Check sheet for the modelled part. Datum: model origin and axes. Units: mm. Face numbers are marked on the shaded views. A direction names the side the tool comes from. Give positions to 0.01 mm unless a question says otherwise; leave off trailing zeros. Order: outer loops, then holes, each group sorted by start corner. A loop starts at its lowest first (then second) coordinate and runs counter-clockwise, first axis right, second up. Notation, with made-up numbers: M 15,29 L 30,29 A27 ccw 30,62 Z; hole C 7,14 d2. An arc over 180 degrees is marked long. Return JSON: item names as keys, results as strings. Group by question number.
from build123d import *

# Parameters (mm, degrees)
F0_W      = 18.5
F0_H      = 20
F1_DEPTH  = 9
F2_W      = 2
F2_H      = 20
F3_DEPTH  = 5
F4_W      = 9.5
F4_H      = 18
F5_DEPTH  = 8
F6_W      = 9.5
F6_H      = 1
F7_DEPTH  = 4
F8_R      = 2
F9_DEPTH  = 25
F11_DEPTH = 20.001
F12_R     = 1.5


with BuildPart() as f1:
    # F0 (on Top) → F1 (new body)
    with BuildSketch(Plane.XY):
        Rectangle(F0_W, F0_H)
    extrude(amount=F1_DEPTH)

    # F2 (on face) → F3 (cut)
    with BuildSketch(Plane(origin=(0, 0, 0), x_dir=(1, 0, 0), z_dir=(0, 0, -1))):
        with Locations((-8.25, 0)):
            Rectangle(F2_W, F2_H)
        with Locations((8.25, 0)):
            Rectangle(F2_W, F2_H)
    extrude(amount=-F3_DEPTH, mode=Mode.SUBTRACT)

    # F4 (on face) → F5 (cut)
    with BuildSketch(Plane.XY.offset(9)):
        Rectangle(F4_W, F4_H)
    extrude(amount=-F5_DEPTH, mode=Mode.SUBTRACT)

    # F6 (on face) → F7 (cut)
    with BuildSketch(Plane.XY.offset(9)):
        with Locations((0, -9.5)):
            Rectangle(F6_W, F6_H)
        with Locations((0, 9.5)):
            Rectangle(F6_W, F6_H)
    extrude(amount=-F7_DEPTH, mode=Mode.SUBTRACT)

    # F8 (on face) → F9 (cut)
    with BuildSketch(Plane.XY.offset(1)):
        Circle(F8_R)
    extrude(amount=-F9_DEPTH, mode=Mode.SUBTRACT)

    # F10 (on face) → F11 (cut, through all)
    with BuildSketch(Plane.XZ.offset(10)):
        Polygon((-9.25, 9), (-9.25, 5), (-7.25, 9), align=None)
        Polygon((7.25, 9), (9.25, 5), (9.25, 9), align=None)
    extrude(amount=-F11_DEPTH, mode=Mode.SUBTRACT)

    # F12
    f12_edges = [f1.edges().sort_by_distance(p)[0] for p in [
        (-4.75, 0, 9),
        (-7.25, 0, 9),
        (4.75, 0, 9),
        (7.25, 0, 9),
    ]]
    fillet(f12_edges, radius=F12_R)


solid = f1.part
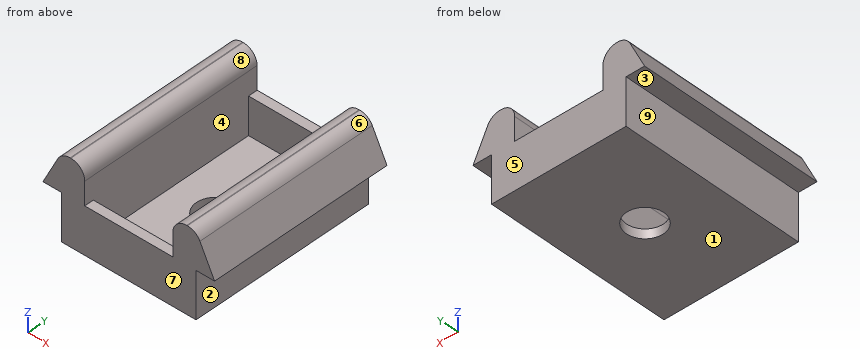
1) Sectioned sample at D-D on z = 2. Record the boundary of the cut face in (x, y), then the cut area to 3 significant figures.
2) Sectioned sample at B-B on z = 6.5. Record the boundary of the cut face in (x, y).
3) Material ranges on line 1 along X through (y, z) = (1.5, 3.75); line 2 along Y through (x, z) = (0, 0.8); line 3 along Y through (x, z) = (0.5, 2), recorded low to high.
4) Sectioned sample at A-A on x = 0. Record the boundary of the cut face in (y, z).
5) Depth check by flat-ended pin: P1, Ø3, axis at y = 2, z = 4, coming from the -X side; P2, Ø0.8, axis at x = 2, y = -9.5, coming from the +Z side; P3, Ø5, axis at y = -1.5, z = 5.5, coming from the +X side. Enter the tip coordinate at first touch or a pass-through.
6) Tool access check on the marked faces 1, 2, 3, 4 and 5. Record the directions out of +Z, -Z, +X, -X, +Y, -Y that give a thin tool (end or side, any length) a straight path to the whole face; none if there is none.
7) Sectioned sample at C-C on y = 0. Record the boundary of the cut face in (x, z), then the cut area to 3 significant figures.
8) Release check for a two-part mould opening along X. For the marked faces 6, 7, 8 and 9 record: released by +X, released by -X, zero draft, split by the parting line, or undercut.
Reply:
{
 "1": {"outline": "M -7.25,-10 L 7.25,-10 L 7.25,10 L -7.25,10 Z; hole M -4.75,-9 L 4.75,-9 L 4.75,9 L -4.75,9 Z", "area": "119 mm^2"},
 "2": {"outline": "M -8.5,-10 L -4.75,-10 L -4.75,10 L -8.5,10 Z; M 4.75,-10 L 8.5,-10 L 8.5,10 L 4.75,10 Z"},
 "3": {"line 1": "-7.25 to -4.75, 4.75 to 7.25", "line 2": "-10 to -2, 2 to 10", "line 3": "-10 to -9, 9 to 10"},
 "4": {"outline": "M -10,0 L -2,0 L -2,1 L -9,1 L -9,5 L -10,5 Z; M 2,0 L 10,0 L 10,5 L 9,5 L 9,1 L 2,1 Z"},
 "5": {"P1": "x = -9.25", "P2": "z = 5", "P3": "x = 9.25"},
 "6": {"face 1": "-Z, +X, -X, +Y, -Y", "face 2": "-Z, +X, +Y, -Y", "face 3": "-Z, -X, +Y, -Y", "face 4": "+Z", "face 5": "+Z, -Z, +X, -X, +Y"},
 "7": {"outline": "M -9.25,5 L -7.25,5 L -7.25,0 L -2,0 L -2,1 L -4.75,1 L -4.75,7.5 A1.5 ccw -6.25,9 L -6.32,9 A1.5 ccw -7.66,8.17 Z; M 2,0 L 7.25,0 L 7.25,5 L 9.25,5 L 7.66,8.17 A1.5 ccw 6.32,9 L 6.25,9 A1.5 ccw 4.75,7.5 L 4.75,1 L 2,1 Z", "area": "57.2 mm^2"},
 "8": {"face 6": "released by +X", "face 7": "zero draft", "face 8": "undercut", "face 9": "released by -X"}
}
